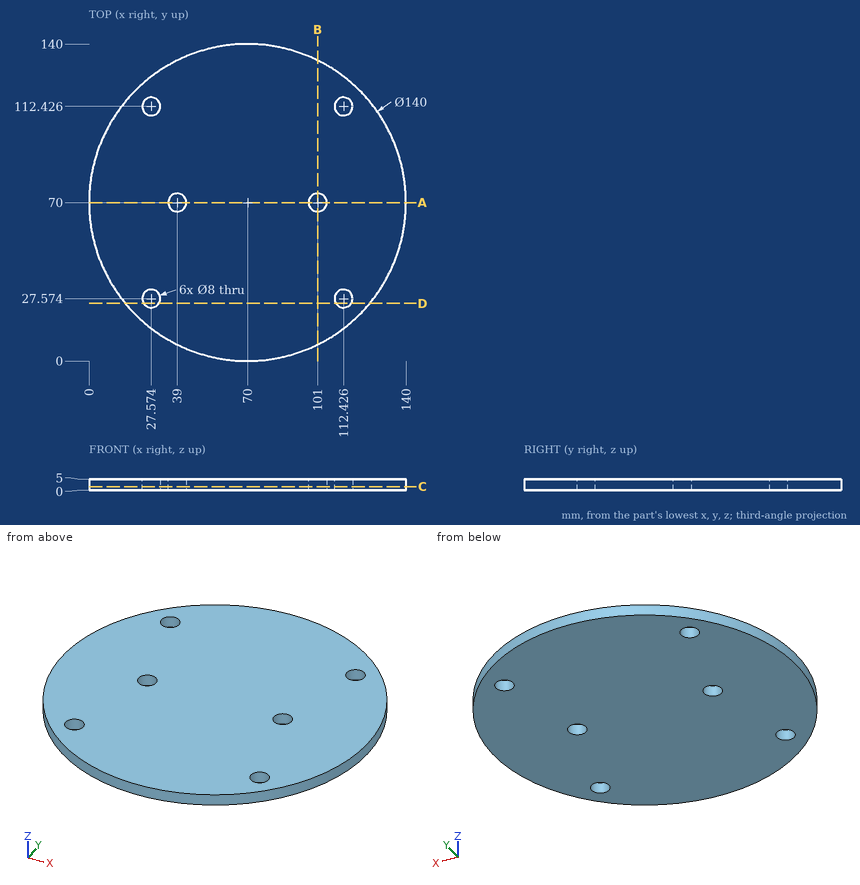
Geometry: see drawing. Coordinates: mm, zero at the bounding-box minimum. Round coordinates to 2 decimals unless told otherwise and drop trailing zeros. Loops run counter-clockwise (first coordinate to the right, second up) from the corner with the lowest first, then second, coordinate; pieces in that order, holes last. Notation, with made-up numbers: M 42.25,39 L 63.25,39 A18 cw 63.25,66 Z; hole C 45,-14 d1. An arc over 180 degrees is marked long. Use a Markdown table: item, result. Add a question column.
1. Line query: line 1 (Y direction, x = 102, z = 2.6); line 2 (Y direction, x = 30.5, z = 1.5) (1 decimal); line 3 (Y direction, x = 39, z = 1.1). Output: solid intervals per line, ascending.
2. Section query A-A on y = 70. Return the cut outline in (x, z).
3. Section query C-C on z = 1.6. Return the cut outline in (x, y), then the cut area to 3 significant figures.
4. Contact query for flat-ended pins moving along their axis: P1, Ø13, axis at x = 27.57, y = 27.57, coming from the +Z side; P2, Ø2, axis at y = 40, z = 4, coming from the -X side; P3, Ø1, axis at y = 122, z = 2, coming from the -X side; P4, Ø6.5, axis at x = 39, y = 70, coming from the +Z side. Output: stop coordinate, or through.
5. Section query B-B on x = 101. Return the cut outline in (y, z).
6. Section query D-D on y = 25.5. Return the cut outline in (x, z) (1 decimal), then the cut area to 3 significant figures.
Reported:
| question | item | result |
|---|---|---|
| 1 | line 1 | y = 7.74 to 66.13, 73.87 to 132.26 |
| 1 | line 2 | y = 12.2 to 24.8, 30.3 to 109.7, 115.2 to 127.8 |
| 1 | line 3 | y = 7.24 to 66, 74 to 132.76 |
| 2 | outline | M 0,0 L 35,0 L 35,5 L 0,5 Z; M 43,0 L 97,0 L 97,5 L 43,5 Z; M 105,0 L 140,0 L 140,5 L 105,5 Z |
| 3 | outline | C 70,70 d140; hole C 27.57,27.57 d8; hole C 27.57,112.43 d8; hole C 39,70 d8; hole C 101,70 d8; hole C 112.43,27.57 d8; hole C 112.43,112.43 d8 |
| 3 | area | 15,100 mm² |
| 4 | P1 | stops at z = 5 |
| 4 | P2 | stops at x = 6.29 |
| 4 | P3 | stops at x = 22.59 |
| 4 | P4 | passes through |
| 5 | outline | M 7.24,0 L 66,0 L 66,5 L 7.24,5 Z; M 74,0 L 132.76,0 L 132.76,5 L 74,5 Z |
| 6 | outline | M 16,0 L 24.2,0 L 24.2,5 L 16,5 Z; M 31,0 L 109,0 L 109,5 L 31,5 Z; M 115.8,0 L 124,0 L 124,5 L 115.8,5 Z |
| 6 | area | 472 mm² |
